from build123d import *
from build123d.topology import SkipClean

# Parameters (mm, degrees)
CUT_EXTRUDE2_REACH = 368.826
CUT_EXTRUDE3_REACH = 388.826
CUT_EXTRUDE3_START = -20


with BuildPart() as part:
    # Sketch1 → Revolve1 (revolve)
    with BuildSketch(Plane(origin=(0, 0, 0), x_dir=(1, 0, 0), z_dir=(0, 1, 0)), mode=Mode.PRIVATE) as revolve1_sk:
        Polygon((52, -44.128440367), (52, 30), (62, 30), (62, 0), (105, -15.779816514), (105, 250), (155, 250), (155, -44.128440367), align=None)
    revolve(revolve1_sk.sketch.rotate(Axis((0, 0, 0), (0, 0, 1)), 180), axis=Axis((0, 0, 0), (0, 0, 1)))

    # Cut-Extrude2: up to this cone (the profile starts outside it)
    with SkipClean():  # the faces are left unmerged after this step: merging them gives an invalid solid
        cut_extrude2_end = Plane(origin=(0, 0, -250), z_dir=(0, 0, 1)).offset(227.247707422) * Cone(2.725e-06, 387.16335, 142.078292578, align=(Align.CENTER, Align.CENTER, Align.MIN), mode=Mode.PRIVATE)
        # Sketch2 → Cut-Extrude2 (cut, up to the surface)
        with BuildSketch(Plane(origin=(0, 0, -250), x_dir=(-1, 0, 0), z_dir=(0, 0, -1)), mode=Mode.PRIVATE) as cut_extrude2_sk1:
            with BuildLine():
                Line((-1.5, 154.992741766), (-1.5, 104.989285168))
                ThreePointArc((-1.5, 104.989285168), (0, 105), (1.5, 104.989285168))
                Line((1.5, 104.989285168), (1.5, 154.992741766))
                ThreePointArc((1.5, 154.992741766), (0, 155), (-1.5, 154.992741766))
            make_face()
        cut_extrude2_tool1 = extrude(cut_extrude2_sk1.sketch, amount=-CUT_EXTRUDE2_REACH, mode=Mode.PRIVATE) - cut_extrude2_end
        add(cut_extrude2_tool1.solids().sort_by_distance((0, 129.997004, -250))[0], mode=Mode.SUBTRACT)
        # Sketch2 → Cut-Extrude2 (cut, up to the surface)
        with BuildSketch(Plane(origin=(0, 0, -250), x_dir=(-1, 0, 0), z_dir=(0, 0, -1)), mode=Mode.PRIVATE) as cut_extrude2_sk2:
            with BuildLine():
                Line((104.989285168, 1.5), (154.992741766, 1.5))
                ThreePointArc((154.992741766, 1.5), (155, 0), (154.992741766, -1.5))
                Line((154.992741766, -1.5), (104.989285168, -1.5))
                ThreePointArc((104.989285168, -1.5), (105, 0), (104.989285168, 1.5))
            make_face()
        cut_extrude2_tool2 = extrude(cut_extrude2_sk2.sketch, amount=-CUT_EXTRUDE2_REACH, mode=Mode.PRIVATE) - cut_extrude2_end
        add(cut_extrude2_tool2.solids().sort_by_distance((-129.997004, 0, -250))[0], mode=Mode.SUBTRACT)
        # Sketch2 → Cut-Extrude2 (cut, up to the surface)
        with BuildSketch(Plane(origin=(0, 0, -250), x_dir=(-1, 0, 0), z_dir=(0, 0, -1)), mode=Mode.PRIVATE) as cut_extrude2_sk3:
            with BuildLine():
                Line((-1.5, -104.989285168), (-1.5, -154.992741766))
                ThreePointArc((-1.5, -154.992741766), (0, -155), (1.5, -154.992741766))
                Line((1.5, -154.992741766), (1.5, -104.989285168))
                ThreePointArc((1.5, -104.989285168), (0, -105), (-1.5, -104.989285168))
            make_face()
        cut_extrude2_tool3 = extrude(cut_extrude2_sk3.sketch, amount=-CUT_EXTRUDE2_REACH, mode=Mode.PRIVATE) - cut_extrude2_end
        add(cut_extrude2_tool3.solids().sort_by_distance((0, -129.997004, -250))[0], mode=Mode.SUBTRACT)
        # Sketch2 → Cut-Extrude2 (cut, up to the surface)
        with BuildSketch(Plane(origin=(0, 0, -250), x_dir=(-1, 0, 0), z_dir=(0, 0, -1)), mode=Mode.PRIVATE) as cut_extrude2_sk4:
            with BuildLine():
                Line((-154.992741766, 1.5), (-104.989285168, 1.5))
                ThreePointArc((-104.989285168, 1.5), (-105, 0), (-104.989285168, -1.5))
                Line((-104.989285168, -1.5), (-154.992741766, -1.5))
                ThreePointArc((-154.992741766, -1.5), (-155, 0), (-154.992741766, 1.5))
            make_face()
        cut_extrude2_tool4 = extrude(cut_extrude2_sk4.sketch, amount=-CUT_EXTRUDE2_REACH, mode=Mode.PRIVATE) - cut_extrude2_end
        add(cut_extrude2_tool4.solids().sort_by_distance((129.997004, 0, -250))[0], mode=Mode.SUBTRACT)

    # Cut-Extrude3: up to this cone (the profile starts outside it)
    with SkipClean():  # the faces are left unmerged after this step: merging them gives an invalid solid
        cut_extrude3_end = Plane(origin=(0, 0, -230), z_dir=(0, 0, 1)).offset(185.943540704) * Cone(2.725e-06, 554.217204308, 203.382459296, align=(Align.CENTER, Align.CENTER, Align.MIN), mode=Mode.PRIVATE)
        # Sketch4 → Cut-Extrude3 (cut, up to the surface)
        with BuildSketch(Plane(origin=(0, 0, -250), x_dir=(-1, 0, 0), z_dir=(0, 0, -1)).offset(CUT_EXTRUDE3_START), mode=Mode.PRIVATE) as cut_extrude3_sk1:
            with BuildLine():
                Line((-154.572798383, -11.5), (-104.368338111, -11.5))
                ThreePointArc((-104.368338111, -11.5), (-74.246212025, -74.246212025), (-11.5, -104.368338111))
                Line((-11.5, -104.368338111), (-11.5, -154.572798383))
                ThreePointArc((-11.5, -154.572798383), (-109.601551084, -109.601551084), (-154.572798383, -11.5))
            make_face()
        cut_extrude3_tool1 = extrude(cut_extrude3_sk1.sketch, amount=-CUT_EXTRUDE3_REACH, mode=Mode.PRIVATE) - cut_extrude3_end
        add(cut_extrude3_tool1.solids().sort_by_distance((85.813767, -85.813767, -230))[0], mode=Mode.SUBTRACT)
        # Sketch4 → Cut-Extrude3 (cut, up to the surface)
        with BuildSketch(Plane(origin=(0, 0, -250), x_dir=(-1, 0, 0), z_dir=(0, 0, -1)).offset(CUT_EXTRUDE3_START), mode=Mode.PRIVATE) as cut_extrude3_sk2:
            with BuildLine():
                Line((11.5, -104.368338111), (11.5, -154.572798383))
                ThreePointArc((11.5, -154.572798383), (109.601551084, -109.601551084), (154.572798383, -11.5))
                Line((154.572798383, -11.5), (104.368338111, -11.5))
                ThreePointArc((104.368338111, -11.5), (74.246212025, -74.246212025), (11.5, -104.368338111))
            make_face()
        cut_extrude3_tool2 = extrude(cut_extrude3_sk2.sketch, amount=-CUT_EXTRUDE3_REACH, mode=Mode.PRIVATE) - cut_extrude3_end
        add(cut_extrude3_tool2.solids().sort_by_distance((-85.813767, -85.813767, -230))[0], mode=Mode.SUBTRACT)
        # Sketch4 → Cut-Extrude3 (cut, up to the surface)
        with BuildSketch(Plane(origin=(0, 0, -250), x_dir=(-1, 0, 0), z_dir=(0, 0, -1)).offset(CUT_EXTRUDE3_START), mode=Mode.PRIVATE) as cut_extrude3_sk3:
            with BuildLine():
                Line((154.572798383, 11.5), (104.368338111, 11.5))
                ThreePointArc((104.368338111, 11.5), (74.246212025, 74.246212025), (11.5, 104.368338111))
                Line((11.5, 104.368338111), (11.5, 154.572798383))
                ThreePointArc((11.5, 154.572798383), (109.601551084, 109.601551084), (154.572798383, 11.5))
            make_face()
        cut_extrude3_tool3 = extrude(cut_extrude3_sk3.sketch, amount=-CUT_EXTRUDE3_REACH, mode=Mode.PRIVATE) - cut_extrude3_end
        add(cut_extrude3_tool3.solids().sort_by_distance((-85.813767, 85.813767, -230))[0], mode=Mode.SUBTRACT)
        # Sketch4 → Cut-Extrude3 (cut, up to the surface)
        with BuildSketch(Plane(origin=(0, 0, -250), x_dir=(-1, 0, 0), z_dir=(0, 0, -1)).offset(CUT_EXTRUDE3_START), mode=Mode.PRIVATE) as cut_extrude3_sk4:
            with BuildLine():
                Line((-11.5, 104.368338111), (-11.5, 154.572798383))
                ThreePointArc((-11.5, 154.572798383), (-109.601551084, 109.601551084), (-154.572798383, 11.5))
                Line((-154.572798383, 11.5), (-104.368338111, 11.5))
                ThreePointArc((-104.368338111, 11.5), (-74.246212025, 74.246212025), (-11.5, 104.368338111))
            make_face()
        cut_extrude3_tool4 = extrude(cut_extrude3_sk4.sketch, amount=-CUT_EXTRUDE3_REACH, mode=Mode.PRIVATE) - cut_extrude3_end
        add(cut_extrude3_tool4.solids().sort_by_distance((85.813767, 85.813767, -230))[0], mode=Mode.SUBTRACT)


solid = part.part
CAD build for the part. Positions are in the model's coordinates, mm. A direction names the side the tool comes from. Round coordinates to 2 decimals unless told otherwise and drop trailing zeros. Use a Markdown table: item, result. Add a question column.
1. Slice it at A-A on z = -16. Give the number of separate pieces and of enclosed holes in the cut face, then the cut area to 3 significant figures.
2. 3-axis set-ups, long thin cutter, end or side, ignore diameter. For faces 1 (the face through (-1.5, 130, -110)), 2 (the face through (84, 84, -230)), 3 (the face through (11.5, -129, -110)), 4 (the face through (104.513, 10.103, -117.73)), 5 (the face through (-83.47, 85.15, -0.3)): which of +Z, -Z, +X, -X, +Y, -Y reach the whole face in a straight line?
3. Pull direction X, two halves, no side cores. Call faces 6 (the face through (10.103, -104.513, -117.73)), 7 (the face through (-85.15, -83.47, -0.3)), 8 (the face through (-130, 1.5, -110)): released by +X, released by -X, zero draft, split by the parting line, or undercut.
4. Flat gauge pins, fed straight in: P1, Ø25, axis at x = 135, z = -80.5, coming from the -Y side; P2, Ø2, axis at x = 20, z = -21, coming from the -Y side; P3, Ø15, axis at x = -131, z = -166.5, coming from the +Y side. Where does each tip first touch, or does it go through?
5. Drill centre lines: probe 1 along X at (y, z) = (-118, -58.5); probe 2 along X at (y, z) = (-3, -154.5). Where is each one in solid material? Low to high.
Reply:
| question | item | result |
|---|---|---|
| 1 | separate pieces | 9 |
| 1 | enclosed holes | 1 |
| 1 | area | 7,590 mm^2 |
| 2 | face 1 | -Z, +Y |
| 2 | face 2 | +X, +Y |
| 2 | face 3 | +X, -Y |
| 2 | face 4 | -Z |
| 2 | face 5 | -X, +Y |
| 3 | face 6 | undercut |
| 3 | face 7 | released by -X |
| 3 | face 8 | zero draft |
| 4 | P1 | stops at y = -11.5 |
| 4 | P2 | stops at y = -59.02 |
| 4 | P3 | stops at y = 11.5 |
| 5 | probe 1 | x = -11.5 to -1.5, 1.5 to 11.5 |
| 5 | probe 2 | x = -154.97 to -104.96, 104.96 to 154.97 |
